The listing builds one solid part. Answer for the finished solid, in the listing's coordinates (mm). Face numbers are marked on the shaded views. A direction names the side the tool comes from. Give positions to 0.01 mm unless a question says otherwise; leave off trailing zeros. Write each loop counter-clockwise with the first axis right and the second up, starting at its lowest first coordinate (ties: lowest second). Pieces come first, ordered by that corner, then holes. Notation, with made-up numbers: (44, 63) - (97, 63) arc R11 cw to (97, 78) - close; hole circle Ø6 at (46, 87.5). An arc over 180 degrees is marked (long way). One line per question, with ' | ' between items. Start each with the question number.
1. A cutting plane is placed at B-B (z = 112). Determine the outline of the cut face in (x, y).
2. A cutting plane is placed at D-D (z = 375). Determine the outline of the cut face in (x, y), then the cut area to 3 significant figures.
3. A cutting plane is placed at C-C (x = 842.5). Determine the outline of the cut face in (y, z).
4. Find the intervals of material crossed by L1, parallel to Y at x = -261, z = 181; L2, parallel to X at y = -171.5, z = 196.5; L3, parallel to X at y = -155.5, z = 162, in increasing order. Write a range as from..to.
5. For the marked faces 4 and 5, determine the directions among +Z, -Z, +X, -X, +Y, -Y from which every point of the face is accessible in a straight line to the end or side of a thin tool.
6. The mould has two halves that part along X. Classify the marked faces 1, 2 and 3: +X half, -X half, draft (parallel to the pull), parting line (faces both ways), or undercut.
7. A cutting plane is placed at A-A (y = -187.5). Determine the outline of the cut face in (x, z), then the cut area to 3 significant figures.
8. Given P1, Ø8, axis at y = -170, z = 347, coming from the +X side; P2, Ø4, axis at y = -106.5, z = 221, coming from the +X side; P3, Ø8, axis at y = -282.5, z = 56, coming from the +X side, each flat-ended and moving along its own axis, determine where each tip first touches the part or whether it passes through.
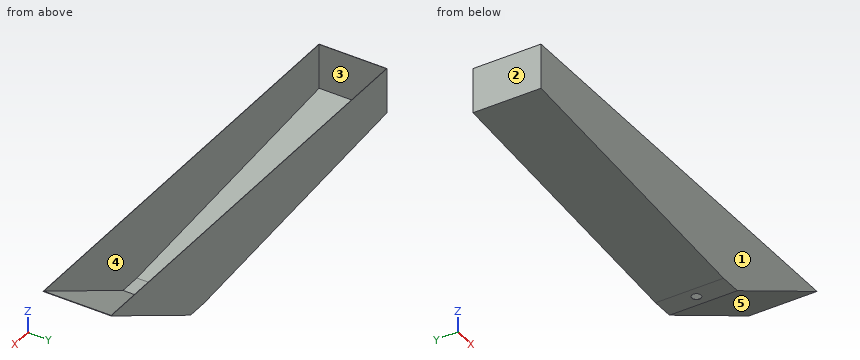
```python
from build123d import *

# Parameters (mm, degrees)
F1_DEPTH = 375
F2_T     = -2
F3_R     = 25
F4_DEPTH = 25


with BuildPart() as f1:
    # F0 (on Front) → F1 (new body)
    with BuildSketch(Plane.XZ):
        Polygon((1321.62507, 399.443237), (-1078.37493, 399.443237), (-1078.37493, 149.443237), (508.828163, 0), (629.769089, 0), align=None)
    extrude(amount=F1_DEPTH)

    # F2
    f2_openings = [f1.faces().sort_by_distance(p)[0] for p in [
        (121.62507, -187.5, 399.443237),
    ]]
    offset(amount=F2_T, openings=f2_openings)

    # F3 (on face) → F4 (cut)
    with BuildSketch(Plane.XY.offset(2)):
        with Locations((569.07765, -187.5)):
            Circle(F3_R)
    extrude(amount=-F4_DEPTH, mode=Mode.SUBTRACT)


solid = f1.part
```
Determined:
1) outline: (-680.7, -375) - (823.76, -375) - (823.76, 0) - (-680.7, 0) - close; hole (-659.36, -373) - (819.76, -373) - (819.76, -2) - (-659.36, -2) - close
2) outline: (-1078.37, -375) - (1279.29, -375) - (1279.29, 0) - (-1078.37, 0) - close; hole (-1076.37, -373) - (1275.29, -373) - (1275.29, -2) - (-1076.37, -2) - close | area: 11,700 mm2
3) outline: (-375, 122.82) - (0, 122.82) - (0, 399.44) - (-2, 399.44) - (-2, 125.13) - (-373, 125.13) - (-373, 399.44) - (-375, 399.44) - close
4) L1: -375..-373, -2..0 | L2: -1078.37..-1076.37, 966.12..970.12 | L3: -1078.37..-1076.37, 906.36..910.36
5) face 4: +Z | face 5: -Z, +X, +Y, -Y
6) face 1: draft | face 2: -X half | face 3: undercut
7) outline: (-1078.37, 149.44) - (508.83, 0) - (544.08, 0) - (544.08, 2) - (508.92, 2) - (-1076.37, 151.26) - (-1076.37, 399.44) - (-1078.37, 399.44) - close; (594.08, 0) - (629.77, 0) - (1321.63, 399.44) - (1317.63, 399.44) - (629.23, 2) - (594.08, 2) - close | area: 5,420 mm2
8) P1: x = 1237.72 | P2: x = 1016.02 | P3: x = 733.69
